Verification items for the finished model (mm, model axes). A direction names the side the tool comes from. Coordinates: 2 decimals unless noted, no trailing zeros. Order: outer loops, then holes, each group sorted by start corner. A loop starts at its lowest first (then second) coordinate and runs counter-clockwise, first axis right, second up.
Q1. Set-up check for faces 4 (the flat face through (70.358, 13, 0)), 5 (the flat face through (-39, 2.464, -5)), 6 (the flat face through (-49.075, 7.656, -0.165)): record each of +Z, -Z, +X, -X, +Y, -Y from which the full face is reachable in a straight line by a thin tool's end or side.
Q2. Cross-section at A-A, the plane y = 20. Record the boundary of the cut face in (x, z) (3 decimals), and give its area (3 significant figures).
Q3. Draft check along Z on faces 1 (the flat face through (-35.16, 10.05, -59.42)), 2 (the flat face through (12, 11, 58.166)), 3 (the flat face through (11, 9, -60.706)). Enter one of: pulls with the +Z half, pulls with the -Z half, needs draft (parallel to the pull), parting line crosses it, or undercut.
Q4. Cross-section at C-C, the plane z = 0. Count the separate pieces of the cut face and the enclosed holes in it, and give its area (3 significant figures).
Q5. Depth check by flat-ended pin: P1, Ø10, axis at y = 14.5, z = 4, coming from the -X side; P2, Ø2.5, axis at y = 4, z = 5, coming from the -X side; P3, Ø12, axis at x = -40.13, z = -6.73, coming from the +Y side. Enter the tip coordinate at first touch or a pass-through.
Q6. Thickness scan on line 1 (Z direction, x = 0, y = 12.5); line 2 (Z direction, x = 45, y = 32); line 3 (Y direction, x = 14.5, z = -11.5). Record the ranges inside material, lowest first.
Q7. Cross-section at B-B, the plane z = 50.5. Record the boundary of the cut face in (x, y).
from build123d import *

# Parameters (mm, degrees)
SKETCH3_W                                       = 90.422573022
SKETCH3_H                                       = 121.412
BOSS_EXTRUDE4_DEPTH                             = 2.54
BOSS_EXTRUDE5_DEPTH                             = 30.48
CUT_EXTRUDE2_DEPTH                              = 122.412
BOSS_EXTRUDE6_DEPTH                             = 33.02
SKETCH9_W                                       = 10.16
SKETCH9_H                                       = 23.622
CUT_EXTRUDE3_DEPTH                              = 27.94
BOSS_EXTRUDE7_DEPTH                             = 2.54
SKETCH12_W                                      = 23.622
SKETCH12_H                                      = 3.81
CUT_EXTRUDE4_DEPTH                              = 10.16
SKETCH13_W                                      = 13.97
SKETCH13_H                                      = 3.81
CUT_EXTRUDE5_DEPTH                              = 13.141913489
BOSS_EXTRUDE9_REACH                             = 62.706
BOSS_EXTRUDE9_DIRECTION_2_REACH                 = 62.706
CBORE_FOR_6_PAN_HEAD_MACHINE_SCREW1_D           = 3.6576
CBORE_FOR_6_PAN_HEAD_MACHINE_SCREW1_CBORE_D     = 7.54126
CBORE_FOR_6_PAN_HEAD_MACHINE_SCREW1_CBORE_DEPTH = 2.4638
F_6_CLEARANCE_HOLE1_D                           = 3.6576
SKETCH21_W                                      = 43.815
SKETCH21_H                                      = 22.86
CUT_EXTRUDE6_DEPTH                              = 33.461913489
CHAMFER1_SIZE                                   = 2.54
CHAMFER2_SIZE                                   = 3.81
SKETCH23_W                                      = 10.16
SKETCH23_H                                      = 23.622
CUT_EXTRUDE8_DEPTH                              = 0.762
CHAMFER3_SIZE                                   = 0.762


with BuildPart() as part:
    # Sketch3 → Boss-Extrude4 (new body)
    with BuildSketch(Plane(origin=(0, 0, 0), x_dir=(1, 0, 0), z_dir=(0, 1, 0))):
        Rectangle(SKETCH3_W, SKETCH3_H)
    extrude(amount=BOSS_EXTRUDE4_DEPTH)

    # Sketch6 → Boss-Extrude5 (add)
    with BuildSketch(Plane(origin=(0, 2.54, 0), x_dir=(1, 0, 0), z_dir=(0, 1, 0))):
        Polygon((45.211286511, -60.706), (45.211286511, 60.706), (-45.211286511, 60.706), (-45.211286511, 58.166), (42.671286511, 58.166), (42.671286511, -58.166), (-45.211286511, -58.166), (-45.211286511, -60.706), align=None)
    extrude(amount=BOSS_EXTRUDE5_DEPTH)

    # Sketch7 → Cut-Extrude2 (cut, through all)
    with BuildSketch(Plane.XY.offset(60.706)):
        Polygon((-42.671286511, 2.54), (-27.431286511, 17.78), (27.431286511, 17.78), (42.671286511, 33.02), (-45.211286511, 33.02), (-45.211286511, 2.54), align=None)
    extrude(amount=-CUT_EXTRUDE2_DEPTH, mode=Mode.SUBTRACT)

    # Sketch8 → Boss-Extrude6 (add)
    with BuildSketch(Plane(origin=(0, 0, 0), x_dir=(1, 0, 0), z_dir=(0, 1, 0))):
        Polygon((45.211286511, 14.351), (71.009871827, 14.351), (74.602950485, 10.757921342), (75.1332, 6.985), (70.358, 6.985), (70.358, -6.985), (75.1332, -6.985), (74.602950485, -10.757921342), (71.009871827, -14.351), (45.211286511, -14.351), align=None)
    extrude(amount=BOSS_EXTRUDE6_DEPTH)

    # Sketch9 → Cut-Extrude3 (cut)
    with BuildSketch(Plane(origin=(0, 33.02, 0), x_dir=(1, 0, 0), z_dir=(0, 1, 0))):
        with Locations((47.751286511, 0)):
            Rectangle(SKETCH9_W, SKETCH9_H)
    extrude(amount=-CUT_EXTRUDE3_DEPTH, mode=Mode.SUBTRACT)

    # Sketch11 → Boss-Extrude7 (add)
    with BuildSketch(Plane(origin=(0, 2.54, 0), x_dir=(1, 0, 0), z_dir=(0, 1, 0))):
        Polygon((35.051286511, 58.166), (27.431286511, 58.166), (29.971286511, 55.626), (32.511286511, 55.626), align=None)
        Polygon((-29.971286511, 55.626), (-32.511286511, 55.626), (-35.051286511, 58.166), (-27.431286511, 58.166), align=None)
        Polygon((29.971286511, -55.626), (32.511286511, -55.626), (35.051286511, -58.166), (27.431286511, -58.166), align=None)
        Polygon((-27.431286511, -58.166), (-29.971286511, -55.626), (-32.511286511, -55.626), (-35.051286511, -58.166), align=None)
    extrude(amount=BOSS_EXTRUDE7_DEPTH)

    # Sketch12 → Cut-Extrude4 (cut)
    with BuildSketch(Plane.ZY.offset(-52.831286511)):
        with Locations((0, 27.305)):
            Rectangle(SKETCH12_W, SKETCH12_H)
    extrude(amount=-CUT_EXTRUDE4_DEPTH, mode=Mode.SUBTRACT)

    # Sketch13 → Cut-Extrude5 (cut, through all)
    with BuildSketch(Plane.ZY.offset(-62.991286511)):
        with Locations((0, 27.305)):
            Rectangle(SKETCH13_W, SKETCH13_H)
    extrude(amount=-CUT_EXTRUDE5_DEPTH, mode=Mode.SUBTRACT)

    # Boss-Extrude9: up to this face of the body (flat: up to its plane)
    boss_extrude9_end = Plane(part.part.faces().sort_by_distance((48.970486511, 20.0406, -11.811))[0])
    # Sketch15 → Boss-Extrude9 (add, up to the picked face)
    with BuildSketch(Plane.XY, mode=Mode.PRIVATE) as boss_extrude9_sk1:
        Polygon((-62.991286511, 10.16), (-52.831286511, 10.16), (-45.211286511, 5.08), (-35.051286511, 5.08), (-35.051286511, 2.54), (-45.211286511, 2.54), (-45.211286511, 0), (-52.831286511, 0), (-52.831286511, 6.35), (-62.991286511, 6.35), align=None)
    boss_extrude9_tool1 = split(extrude(boss_extrude9_sk1.sketch, amount=-BOSS_EXTRUDE9_REACH, mode=Mode.PRIVATE), bisect_by=boss_extrude9_end, keep=Keep.BOTH, mode=Mode.PRIVATE)
    add(boss_extrude9_tool1.solids().sort_by_distance((-50.157602, 5.280526, 0))[0])

    # Boss-Extrude9 direction 2: up to this face of the body (flat: up to its plane)
    boss_extrude9_direction_2_end = Plane(part.part.faces().sort_by_distance((48.970486511, 20.0406, 11.811))[0])
    # Sketch15 → Boss-Extrude9 direction 2 (add, up to the picked face)
    with BuildSketch(Plane.XY, mode=Mode.PRIVATE) as boss_extrude9_direction_2_sk1:
        Polygon((-62.991286511, 10.16), (-52.831286511, 10.16), (-45.211286511, 5.08), (-35.051286511, 5.08), (-35.051286511, 2.54), (-45.211286511, 2.54), (-45.211286511, 0), (-52.831286511, 0), (-52.831286511, 6.35), (-62.991286511, 6.35), align=None)
    boss_extrude9_direction_2_tool1 = split(extrude(boss_extrude9_direction_2_sk1.sketch, amount=BOSS_EXTRUDE9_DIRECTION_2_REACH, mode=Mode.PRIVATE), bisect_by=boss_extrude9_direction_2_end, keep=Keep.BOTH, mode=Mode.PRIVATE)
    add(boss_extrude9_direction_2_tool1.solids().sort_by_distance((-50.157602, 5.280526, 0))[0])

    # CBORE for #6 Pan Head Machine Screw1 (through all)
    with Locations(Plane(origin=(0, 0, 0), x_dir=(-1, 0, 0), z_dir=(0, -1, 0))):
        with Locations((-47.751286511, 6.731), (-47.751286511, -6.731), (40.131286511, 6.731), (40.131286511, -6.731)):
            CounterBoreHole(CBORE_FOR_6_PAN_HEAD_MACHINE_SCREW1_D / 2, CBORE_FOR_6_PAN_HEAD_MACHINE_SCREW1_CBORE_D / 2, CBORE_FOR_6_PAN_HEAD_MACHINE_SCREW1_CBORE_DEPTH)

    # #6 Clearance Hole1 (through all)
    with Locations(Plane(origin=(0, 33.02, 0), x_dir=(1, 0, 0), z_dir=(0, 1, 0))):
        with Locations((-57.911286511, 0), (57.911286511, 0)):
            Hole(F_6_CLEARANCE_HOLE1_D / 2)

    # Sketch21 → Cut-Extrude6 (cut, through all)
    with BuildSketch(Plane.ZY.offset(-42.671286511)):
        with Locations((-36.2585, 17.78)):
            Rectangle(SKETCH21_W, SKETCH21_H)
        with Locations((36.2585, 17.78)):
            Rectangle(SKETCH21_W, SKETCH21_H)
    extrude(amount=-CUT_EXTRUDE6_DEPTH, mode=Mode.SUBTRACT)

    # Chamfer1
    chamfer1_edges = [part.edges().sort_by_distance(p)[0] for p in [
        (-52.831286511, 0, 0),
        (-35.051286511, 3.81, -11.811),
        (-62.991286511, 8.255, -11.811),
        (-62.991286511, 8.255, 11.811),
        (-35.051286511, 3.81, 11.811),
    ]]
    chamfer(chamfer1_edges, length=CHAMFER1_SIZE)

    # Chamfer2
    chamfer2_edges = [part.edges().sort_by_distance(p)[0] for p in [
        (45.211286511, 3.175, -14.351),
        (45.211286511, 3.175, 14.351),
        (45.211286511, 31.115, -14.351),
        (45.211286511, 31.115, 14.351),
    ]]
    chamfer(chamfer2_edges, length=CHAMFER2_SIZE)

    # Sketch23 → Cut-Extrude8 (cut)
    with BuildSketch(Plane.XZ.offset(-6.35)):
        with Locations((-57.911286511, 0)):
            Rectangle(SKETCH23_W, SKETCH23_H)
    extrude(amount=-CUT_EXTRUDE8_DEPTH, mode=Mode.SUBTRACT)

    # Chamfer3
    chamfer3_edges = [part.edges().sort_by_distance(p)[0] for p in [
        (-62.991286511, 10.16, 0),
        (-62.991286511, 7.112, 0),
    ]]
    chamfer(chamfer3_edges, length=CHAMFER3_SIZE)


solid = part.part
Check values:
1. face 4: +X, +Y, -Y
1. face 5: -Y
1. face 6: +Z, -Z, +Y
2. outline: (29.651, -60.706) - (45.211, -60.706) - (45.211, -58.166) - (29.651, -58.166) - close; (29.651, 58.166) - (45.211, 58.166) - (45.211, 60.706) - (29.651, 60.706) - close; (42.671, -14.351) - (71.01, -14.351) - (74.603, -10.758) - (75.133, -6.985) - (70.358, -6.985) - (70.358, 6.985) - (75.133, 6.985) - (74.603, 10.758) - (71.01, 14.351) - (42.671, 14.351) - (42.671, 11.811) - (52.831, 11.811) - (52.831, -11.811) - (42.671, -11.811) - close; hole circle Ø3.658 at (57.911, 0)
2. area: 675 mm2
3. face 1: needs draft
3. face 2: undercut
3. face 3: pulls with the -Z half
4. separate pieces: 5
4. enclosed holes: 0
4. area: 780 mm2
5. P1: stops at x = -62.89
5. P2: stops at x = -52.83
5. P3: stops at y = 5.69
6. line 1: z = -60.71 to -58.17, 58.17 to 60.71
6. line 2: z = -60.71 to -11.81, 11.81 to 60.71
6. line 3: y = 0 to 2.54
7. outline: (-45.21, 0) - (45.21, 0) - (45.21, 6.35) - (42.67, 6.35) - (42.67, 2.54) - (-45.21, 2.54) - close; (42.67, 29.21) - (45.21, 29.21) - (45.21, 33.02) - (42.67, 33.02) - close
